Model file for the job. Use its own axes, mm. A direction names the side the tool comes from. Give positions to 0.01 mm unless a question says otherwise; leave off trailing zeros. Order: outer loops, then holes, each group sorted by start corner. A loop starts at its lowest first (then second) coordinate and runs counter-clockwise, first axis right, second up. Notation, with made-up numbers: (88.25, 14) -> (135.25, 14) arc R31 ccw to (135.25, 48) -> close; hole circle Ø1 at (-5.5, 27). An arc over 180 degrees is marked (long way). Use CSV: the item, a comma, the result in double quotes. Start each with the question number.
1. 3-axis set-ups, long thin cutter, end or side, ignore diameter. For faces 1 (the flat face through (-3.131, 59.48, -5.525)), 2 (the cylindrical face through (-1.468, 6.261, 1.915)): which of +Z, -Z, +X, -X, +Y, -Y reach the whole face in a straight line?
2. Cut at B-B on z = -5. List the corners of the cut face in (x, y).
3. Pull direction Z, two halves, no side cores. Call faces 3 (the flat face through (-2, 12.7, 1)), 4 (the flat face through (3.131, 59.48, 5.525)), 5 (the flat face through (-6.35, 59, 0)): released by +Z, released by -Z, zero draft, split by the parting line, or undercut.
4. Cut at C-C on x = 4.25. List the corners of the cut face in (y, z), then the cut area to 3 significant figures.
5. Wall check: line 1 (Z direction, x = 0, y = 15.2); line 2 (X direction, y = 9.75, z = 0); line 3 (X direction, y = 15.5, z = 0). Give the ranges that are in metal, low to high. Write a range as from..to.
6. Cut at A-A on y = 65. List the corners of the cut face in (x, z).
7. Drop flat-ended pins along their axis: pin 1 (6 mm diameter, centred on x = 4.5, z = 2, fed in from -Y); pin 2 (2 mm diameter, centred on y = 103.5, z = 5.5, fed in from +X). Give the stop position or say it passes through.
```python
from build123d import *

# Parameters (mm, degrees)
BOSS_EXTRUDE1_DEPTH              = 120.65
F_10_32_TAPPED_HOLE1_D           = 4.0386
F_10_32_TAPPED_HOLE1_DEPTH       = 16.764
F_10_32_TAPPED_HOLE1_CBORE_D     = 4.826
F_10_32_TAPPED_HOLE1_CBORE_DEPTH = 12.7
F_10_32_TAPPED_HOLE1_TIP         = 1.213317848


with BuildPart() as part:
    # Sketch1 → Boss-Extrude1 (new body)
    with BuildSketch(Plane(origin=(0, 0, 0), x_dir=(1, 0, 0), z_dir=(0, 1, 0))):
        Polygon((0, 7.332348419), (-6.35, 3.666174209), (-6.35, -3.666174209), (0, -7.332348419), (6.35, -3.666174209), (6.35, 3.666174209), align=None)
    extrude(amount=BOSS_EXTRUDE1_DEPTH)

    # #10-32 Tapped Hole1
    with Locations(Plane(origin=(0, 0, 0), x_dir=(0, 0, -1), z_dir=(0, -1, 0))):
        with Locations((0, 0)):
            CounterBoreHole(F_10_32_TAPPED_HOLE1_D / 2, F_10_32_TAPPED_HOLE1_CBORE_D / 2, F_10_32_TAPPED_HOLE1_CBORE_DEPTH, depth=F_10_32_TAPPED_HOLE1_DEPTH)
            with Locations((0, 0, -(F_10_32_TAPPED_HOLE1_DEPTH + F_10_32_TAPPED_HOLE1_TIP / 2))):  # 118° drill point
                Cone(0, F_10_32_TAPPED_HOLE1_D / 2, F_10_32_TAPPED_HOLE1_TIP, mode=Mode.SUBTRACT)


solid = part.part
```
Verdict:
1,face 1,"-Z, -X, +Y, -Y"
1,face 2,"-Y"
2,outline,"(-4.04, 0) -> (4.04, 0) -> (4.04, 120.65) -> (-4.04, 120.65) -> close"
3,face 3,"undercut"
3,face 4,"released by +Z"
3,face 5,"zero draft"
4,outline,"(0, -4.88) -> (120.65, -4.88) -> (120.65, 4.88) -> (0, 4.88) -> close"
4,area,"1,180 mm^2"
5,line 1,"-7.33..-2.02, 2.02..7.33"
5,line 2,"-6.35..-2.41, 2.41..6.35"
5,line 3,"-6.35..-2.02, 2.02..6.35"
6,outline,"(-6.35, -3.67) -> (0, -7.33) -> (6.35, -3.67) -> (6.35, 3.67) -> (0, 7.33) -> (-6.35, 3.67) -> close"
7,pin 1,"y = 0"
7,pin 2,"x = 4.91"
